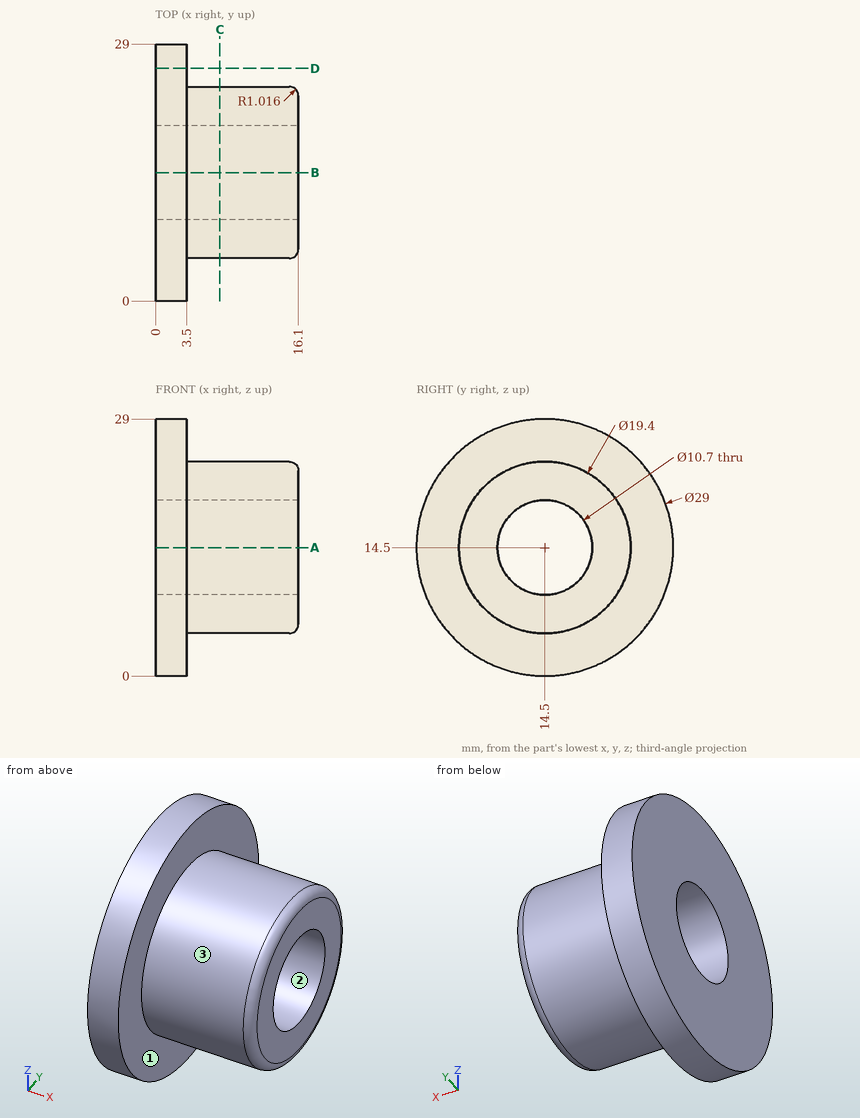
The figure shows three views and two pictorial views of one solid part (mm, origin at its lowest corner). Answer the questions. Coordinates: 2 decimals unless noted, no trailing zeros. Write each loop counter-clockwise with the first axis right and the second up, starting at its lowest first coordinate (ties: lowest second). Pieces come first, ordered by that corner, then holes.
1. Flat-ended cylindrical pins translate along their axes: pin 1 (3 mm diameter, centred on x = 11.5, y = 22, fed in from -Z); pin 2 (2 mm diameter, centred on y = 17.5, z = 11, fed in from +X); pin 3 (2 mm diameter, centred on y = 3.5, z = 7.5, fed in from +X); pin 4 (1.5 mm diameter, centred on x = 6.5, y = 9, fed in from -Z). Find the tip coordinate at first contact, or state that the pin passes through.
Results list:
pin 1: stops at z = 6.88
pin 2: stops at x = 16.1
pin 3: stops at x = 3.5
pin 4: stops at z = 6.04
2. Consider line 1 along Y through (x, z) = (8.25, 14.5); line 2 along X through (y, z) = (2.75, 10). Determine where each line is inside the solid, lowest interval first.
Results list:
line 1: y = 4.8 to 9.15, 19.85 to 24.2
line 2: x = 0 to 3.5
3. The part is cut by section A-A, the plane z = 14.5. Write down the section's boundary in (x, y), and give its area (3 significant figures).
Results list:
outline: (0, 0) - (3.5, 0) - (3.5, 4.8) - (15.08, 4.8) arc R1.02 ccw to (16.1, 5.82) - (16.1, 9.15) - (0, 9.15) - close; (0, 19.85) - (16.1, 19.85) - (16.1, 23.18) arc R1.02 ccw to (15.08, 24.2) - (3.5, 24.2) - (3.5, 29) - (0, 29) - close
area: 173 mm2
4. The part is cut by section D-D, the plane y = 26.25. Write down the section's boundary in (x, z).
Results list:
outline: (0, 6) - (3.5, 6) - (3.5, 23) - (0, 23) - close
5. For a pull along Z with two mould halves and no side action, classify the marked faces 1, 2 and 3 as +Z half, -Z half, draft (parallel to the pull), parting line (faces both ways), or undercut.
Results list:
face 1: draft
face 2: undercut
face 3: parting line
6. The part is cut by section C-C, the plane x = 7.25. Write down the section's boundary in (y, z).
Results list:
outline: circle Ø19.4 at (14.5, 14.5); hole circle Ø10.7 at (14.5, 14.5)
